The model under review builds one solid part; all positions refer to its coordinate system, in mm. Face numbers are marked on the shaded views. A direction names the side the tool comes from. Coordinates: 2 decimals unless noted, no trailing zeros. Write each loop counter-clockwise with the first axis right and the second up, starting at its lowest first coordinate (ties: lowest second). Pieces come first, ordered by that corner, then holes. Notation, with made-up numbers: (45, 7.5) - (68, 7.5) arc R9 cw to (68, 13.5) - close; hole circle Ø2 at (43.25, -21). An arc over 180 degrees is marked (long way). Put each result on its own line as item: value.
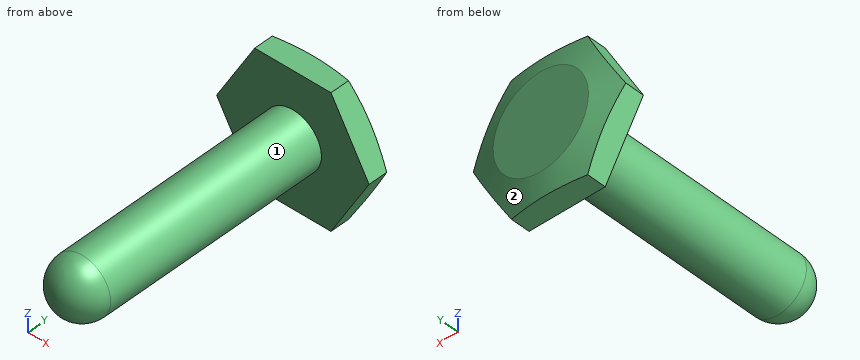
from build123d import *

# Parameters (mm, degrees)
SKETCH2_OUTSIDE_W = 76.662
SKETCH2_OUTSIDE_H = 76.662
HEX_CUT_DEPTH     = 102.798244091


with BuildPart() as part:
    # Sketch1 → Pin Base (revolve)
    with BuildSketch(Plane.XY, mode=Mode.PRIVATE) as pin_base_sk:
        with BuildLine():
            Line((0, 0), (0, -95.25))
            ThreePointArc((0, -95.25), (6.735192091, -92.460192091), (9.525, -85.725))
            Line((9.525, -85.725), (9.525, -9.525))
            Line((9.525, -9.525), (25.4, -9.525))
            Line((25.4, -9.525), (25.4, -3.175))
            Line((25.4, -3.175), (15.875, 0))
            Line((15.875, 0), (0, 0))
        make_face()
    revolve(pin_base_sk.sketch.rotate(Axis((0, 0, 0), (0, -1, 0)), 90), axis=Axis((0, 0, 0), (0, -1, 0)))

    # Sketch2 outside → Hex Cut (cut, through all)
    with BuildSketch(Plane(origin=(0, 0, 0), x_dir=(1, 0, 0), z_dir=(0, 1, 0))):
        Rectangle(SKETCH2_OUTSIDE_W, SKETCH2_OUTSIDE_H)
        Polygon((25.4, 0), (12.7, 21.997045256), (-12.7, 21.997045256), (-25.4, 0), (-12.7, -21.997045256), (12.7, -21.997045256), align=None, mode=Mode.SUBTRACT)
    extrude(amount=-HEX_CUT_DEPTH, mode=Mode.SUBTRACT)


solid = part.part
1. Consider section A-A on x = 0. State the section outline as (y, z) points (3 decimals), plus the area to 3 significant figures.
Determined:
outline: (-85.725, -9.525) - (-9.525, -9.525) - (-9.525, -21.997) - (-2.041, -21.997) - (0, -15.875) - (0, 15.875) - (-2.041, 21.997) - (-9.525, 21.997) - (-9.525, 9.525) - (-85.725, 9.525) arc R9.525 ccw to start
area: 2,000 mm^2
2. For pin 1 Ø2 at (y, z) = (-63, 4.5) entering from +X; pin 2 Ø8 at (y, z) = (-22.5, -7.5) entering from -X; pin 3 Ø10 at (y, z) = (-65, 0) entering from +X (3 decimals); pin 4 Ø5 at (x, z) = (2, 8.5) entering from +Y, all flat-tipped, find the tip position at first contact; note any pin that passes through.
Determined:
pin 1: stops at x = 8.86
pin 2: stops at x = -8.86
pin 3: stops at x = 9.525
pin 4: stops at y = 0
3. Machinability: for the marked faces 1 and 2, which of the approach directions +Z, -Z, +X, -X, +Y, -Y give a long, thin tool a straight path to every point of the face, cutting with its end or side? Answer none if there is none.
Determined:
face 1: -Y
face 2: +Y
4. To check wall thickness, follow probe 1 along Y at (x, z) = (-9, 6.5) (3 decimals); probe 2 along Z at (x, y) = (6, -31); probe 3 along Z at (x, y) = (21.5, -7.5) (3 decimals). State the ranges of each line that lie inside material, in increasing order.
Determined:
probe 1: y = -9.525 to 0
probe 2: z = -7.4 to 7.4
probe 3: z = -6.755 to 6.755
5. Consider section B-B on y = -58.5. State the section outline as (x, z) points (3 decimals), plus the area to 3 significant figures.
Determined:
outline: circle Ø19.05 at (0, 0)
area: 285 mm^2
